```python
from build123d import *

# Parameters (mm, degrees)
F1_DEPTH = 6.35
F3_DEPTH = 38.1
F5_DEPTH = 76.2
F6_W     = 38.1
F6_H     = 12.7
F7_DEPTH = 25.4


with BuildPart() as f1:
    # F0 (on Front) → F1 (new body, symmetric)
    with BuildSketch(Plane.XZ):
        Polygon((-38.934134, 25.4), (-38.934134, 0), (37.265866, 0), (37.265866, 25.4), (11.865866, 50.8), (-13.534134, 50.8), align=None)
    extrude(amount=F1_DEPTH, both=True)

    # F2 (on face) → F3 (join)
    with BuildSketch(Plane.XZ.offset(6.35)):
        Polygon((0, 38.1), (-38.934134, 0), (37.265866, 0), align=None)
    extrude(amount=F3_DEPTH)

    # F4 (on face) → F5 (cut)
    with BuildSketch(Plane.YZ.offset(37.265866)):
        Polygon((-44.45, 38.1), (-44.45, 0), (-6.35, 38.1), align=None)
    extrude(amount=-F5_DEPTH, mode=Mode.SUBTRACT)

    # F6 (on face) → F7 (cut)
    with BuildSketch(Plane(origin=(0, 0, 0), x_dir=(1, 0, 0), z_dir=(0, 0, -1))):
        with Locations((-0.28891, 38.1)):
            Rectangle(F6_W, F6_H)
    extrude(amount=-F7_DEPTH, mode=Mode.SUBTRACT)


solid = f1.part
```
Part model, mm, in its own coordinate system. A direction names the side the tool comes from. Round coordinates to 2 decimals unless told otherwise and drop trailing zeros. Write each loop counter-clockwise with the first axis right and the second up, starting at its lowest first coordinate (ties: lowest second). Pieces come first, ordered by that corner, then holes.
Item 1: Cut at B-B, the plane z = 7. Give the cut face in (x, y), plus the area to 3 significant figures.
Results:
outline: (-38.93, -6.35) - (-31.78, -6.35) - (-31.78, -37.45) - (-19.34, -37.45) - (-19.34, -31.75) - (18.76, -31.75) - (18.76, -37.45) - (30.42, -37.45) - (30.42, -6.35) - (37.27, -6.35) - (37.27, 6.35) - (-38.93, 6.35) - close
area: 2,680 mm2
Item 2: Cut at C-C, the plane x = 10.5. Give the cut face in (y, z), plus the area to 3 significant figures.
Results:
outline: (-31.75, 0) - (6.35, 0) - (6.35, 50.8) - (-6.35, 50.8) - (-6.35, 27.36) - (-17.09, 27.36) - (-31.75, 12.7) - close
area: 1,230 mm2
Item 3: Two-plate mould, pull along X, no slides. Class faces 4 (the flat face through (-26.056, -0.089, 38.278)), 5 (the flat face through (-19.339, -37, 5)), 6 (the flat face through (37.266, 0, 13)): +X half, -X half, draft (parallel to the pull), parting line (faces both ways), or undercut.
Results:
face 4: -X half
face 5: undercut
face 6: +X half
Item 4: Cut at A-A, the plane y = -36. Give the cut face in (x, z).
Results:
outline: (-38.93, 0) - (-19.34, 0) - (-19.34, 8.45) - (-30.3, 8.45) - close; (18.76, 0) - (37.27, 0) - (29, 8.45) - (18.76, 8.45) - close
Item 5: Drop flat-ended pins along their axis: pin 1 Ø10 at (y, z) = (-40.5, 9) entering from +X; pin 2 Ø8 at (x, y) = (3, -16) entering from +Z; pin 3 Ø10 at (x, z) = (-5, 7) entering from -Y. Give the stop position or say it passes through.
Results:
pin 1: stops at x = 33.35
pin 2: stops at z = 32.45
pin 3: stops at y = -31.75
Item 6: Cut at D-D, the plane y = 1.5. Give the cut face in (x, z).
Results:
outline: (-38.93, 0) - (37.27, 0) - (37.27, 25.4) - (11.87, 50.8) - (-13.53, 50.8) - (-38.93, 25.4) - close
Item 7: Which spindle directions (+Z, -Z, +X, -X, +Y, -Y) get a long thin tool onto all of the face, cutting with end or side? Do faces 1 (the flat face through (-1.4, -6.35, 37)), 2 (the flat face through (23.034, -20.9, 14.55)), 3 (the flat face through (18.761, -37, 5)). Say none if no direction does.
Results:
face 1: +Z, -Y
face 2: +Z, +X, -Y
face 3: +Z, -Z, -Y
Item 8: Probe L1, parallel to Y at x = -21, z = 21; L2, parallel to X at y = -6, z = 39.5; L3, parallel to Z at x = -6, y = -7. List the from-to ranges inside material, lowest first.
Results:
L1: y = -6.35 to 6.35
L2: x = -24.83 to 23.17
L3: z = 0 to 32.23
